Answer from the drawing. Dimensions are ordinates in mm from the lowest x, y and z of the part. Give positions to 0.01 mm unless a question says otherwise; leave off trailing zeros. Order: outer loops, then holes, each group sorted by start corner. A loop starts at its lowest first (then second) coordinate and runs counter-clockwise, first axis right, second up. Notation, with made-up numbers: (13, 49.5) -> (51, 49.5) arc R17 ccw to (51, 78.5) -> close; hole circle Ø1 at (-28, -7.75). An arc over 180 degrees is marked (long way). Answer as a JSON object with one key per item and string values. Group by question number.
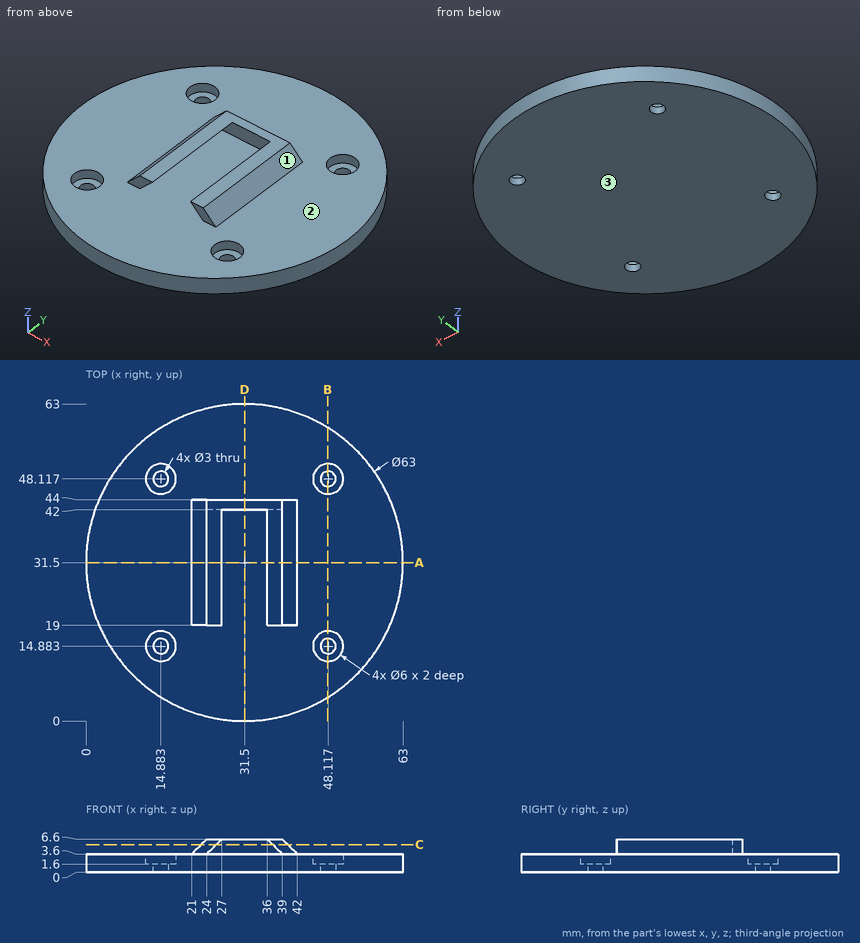
(1) A cutting plane is placed at D-D (x = 31.5). Determine the outline of the cut face in (y, z), and give its area (3 significant figures).
(2) A cutting plane is placed at C-C (z = 5.5). Determine the outline of the cut face in (x, y).
(3) Find the intervals of material crossed by line 1 along X through (y, z) = (50.5, 3.5); line 2 along Y through (x, z) = (29.5, 3.75), in increasing order. Write a range as [from, to].
(4) For a pull along X with two mould halves and no side action, classify the marked faces 1, 2 and 3 as +X half, -X half, draft (parallel to the pull), parting line (faces both ways), or undercut.
(5) A cutting plane is placed at A-A (y = 31.5). Determine the outline of the cut face in (x, z), and give its area (3 significant figures).
(6) A cutting plane is placed at B-B (x = 48). Determine the outline of the cut face in (y, z), and give its area (3 significant figures).
(7) Flat-ended cylindrical pins translate along their axes: pin 1 Ø5 at (x, y) = (24.5, 52) entering from -Z; pin 2 Ø3 at (x, y) = (49, 47.5) entering from +Z; pin 3 Ø12 at (x, y) = (44.5, 54) entering from +Z; pin 4 Ø0.9 at (x, z) = (28.5, 5.5) entering from +Y. Find the tip coordinate at first contact, or state that the pin passes through.
Check sheet entries:
{
 "1": {"outline": "(0, 0) -> (63, 0) -> (63, 3.6) -> (44, 3.6) -> (44, 6.6) -> (42, 6.6) -> (42, 3.6) -> (0, 3.6) -> close", "area": "233 mm2"},
 "2": {"outline": "(22.9, 19) -> (25.9, 19) -> (25.9, 42) -> (37.1, 42) -> (37.1, 19) -> (40.1, 19) -> (40.1, 44) -> (22.9, 44) -> close"},
 "3": {"line 1": "x = [6.38, 13.06], [16.71, 46.29], [49.94, 56.62]", "line 2": "y = [42, 44]"},
 "4": {"face 1": "+X half", "face 2": "undercut", "face 3": "draft"},
 "5": {"outline": "(0, 0) -> (63, 0) -> (63, 3.6) -> (42, 3.6) -> (39, 6.6) -> (36, 6.6) -> (39, 3.6) -> (24, 3.6) -> (27, 6.6) -> (24, 6.6) -> (21, 3.6) -> (0, 3.6) -> close", "area": "245 mm2"},
 "6": {"outline": "(4.67, 0) -> (13.39, 0) -> (13.39, 1.6) -> (11.89, 1.6) -> (11.89, 3.6) -> (4.67, 3.6) -> close; (16.38, 0) -> (46.62, 0) -> (46.62, 1.6) -> (45.12, 1.6) -> (45.12, 3.6) -> (17.88, 3.6) -> (17.88, 1.6) -> (16.38, 1.6) -> close; (49.61, 0) -> (58.33, 0) -> (58.33, 3.6) -> (51.11, 3.6) -> (51.11, 1.6) -> (49.61, 1.6) -> close", "area": "160 mm2"},
 "7": {"pin 1": "stops at z = 0", "pin 2": "stops at z = 1.6", "pin 3": "stops at z = 3.6", "pin 4": "stops at y = 44"}
}
